```python
from build123d import *

# Parameters (mm, degrees)
SKETCH1_R               = 39.3
SKETCH1_R_2             = 38.15
BOSS_EXTRUDE1_DEPTH     = 120
CUT_EXTRUDE1_REACH      = 154.977
CUT_EXTRUDE1_END_RADIUS = 38.15
SKETCH2_R               = 3.55
CIRPATTERN1_COUNT       = 4


with BuildPart() as part:
    # Sketch1 → Boss-Extrude1 (new body)
    with BuildSketch(Plane(origin=(0, 0, 0), x_dir=(1, 0, 0), z_dir=(0, 1, 0))):
        with Locations(Location((0, 0, 0), (0, 0, 270))):
            Circle(SKETCH1_R)
        with Locations(Location((0, 0, 0), (0, 0, 270))):
            Circle(SKETCH1_R_2, mode=Mode.SUBTRACT)
    extrude(amount=BOSS_EXTRUDE1_DEPTH)

    # Cut-Extrude1: up to this cylinder (the profile starts outside it)
    cut_extrude1_end = Plane(origin=(0, 25, 0), z_dir=(0, -1, 0)) * Cylinder(CUT_EXTRUDE1_END_RADIUS, 387.254, mode=Mode.PRIVATE)
    # Sketch2 → Cut-Extrude1 (cut, up to the surface)
    with BuildSketch(Plane(origin=(-27.789296501, 0, -27.789296501), x_dir=(0, -1, 0), z_dir=(-0.7071067811865464, 0, -0.7071067811865488)), mode=Mode.PRIVATE) as cut_extrude1_sk1:
        with Locations(Location((-25, 0, 0), (0, 0, 90))):
            Circle(SKETCH2_R)
    cut_extrude1_tool1 = extrude(cut_extrude1_sk1.sketch, amount=-CUT_EXTRUDE1_REACH, mode=Mode.PRIVATE) - cut_extrude1_end
    cut_extrude1 = cut_extrude1_tool1.solids().sort_by_distance((-27.789297, 25, -27.789297))[0]
    add(cut_extrude1, mode=Mode.SUBTRACT)

    # CirPattern1: Cut-Extrude1 ×4 about axis
    cirpattern1_axis = Axis((0, 120, 0), (0, -1, 0))
    for i in range(1, CIRPATTERN1_COUNT):
        add(cut_extrude1.rotate(cirpattern1_axis, i * 360 / CIRPATTERN1_COUNT), mode=Mode.SUBTRACT)


solid = part.part
```
Geometry check sheet. Reference: the model listing, model coordinates, mm. Coordinates: 2 decimals unless noted, no trailing zeros. Write each loop counter-clockwise with the first axis right and the second up, starting at its lowest first coordinate (ties: lowest second). Pieces come first, ordered by that corner, then holes. Notation, with made-up numbers: M 87,5 L 96,5 A17 cw 96,27 Z; hole C 52,-36.75 d1. An arc over 180 degrees is marked long. Use one line per item in the form item = value. Start each with the question number.
1) Go/stop test with flat-tipped pins: pin 1 Ø5 at (x, y) = (-5.5, 70.5) entering from +Z; pin 2 Ø6 at (x, y) = (-24, 107) entering from +Z; pin 3 Ø1.5 at (x, y) = (-27, 85) entering from -Z. Record where each tip stops, or that it passes through.
2) Thickness scan on probe 1 along X at (y, z) = (78, 0); probe 2 along X at (y, z) = (84, -34); probe 3 along Z at (x, y) = (-9, 56). Record the ranges inside material, lowest first. Write a range as from..to.
3) Section check C-C on y = 81.5. Enter the section's corners in (x, z).
4) Release check for a two-part mould opening along Y. For faces 1 (the flat face through (38, 120, -6)), 2 (the flat face through (38, 0, -6)), 3 (the cylindrical face through (27, 28.52, 27.66)) record: pulls with the +Y half, pulls with the -Y half, needs draft (parallel to the pull), parting line crosses it, or undercut.
5) Section check B-B on x = 0. Enter the section's corners in (y, z).
6) Section check A-A on z = 0. Enter the section's corners in (x, y), and give its area (3 significant figures).
Responses:
q1.pin_1 = 39.19
q1.pin_2 = 33.22
q1.pin_3 = -29.25
q2.probe_1 = -39.3..-38.15, 38.15..39.3
q2.probe_2 = -19.71..-17.3, 17.3..19.71
q2.probe_3 = -38.26..-37.07, 37.07..38.26
q3.outline = C 0,0 d78.6; hole C 0,0 d76.3
q4.face_1 = pulls with the +Y half
q4.face_2 = pulls with the -Y half
q4.face_3 = undercut
q5.outline = M 0,-39.3 L 120,-39.3 L 120,-38.15 L 0,-38.15 Z; M 0,38.15 L 120,38.15 L 120,39.3 L 0,39.3 Z
q6.outline = M -39.3,0 L -38.15,0 L -38.15,120 L -39.3,120 Z; M 38.15,0 L 39.3,0 L 39.3,120 L 38.15,120 Z
q6.area = 276 mm2
